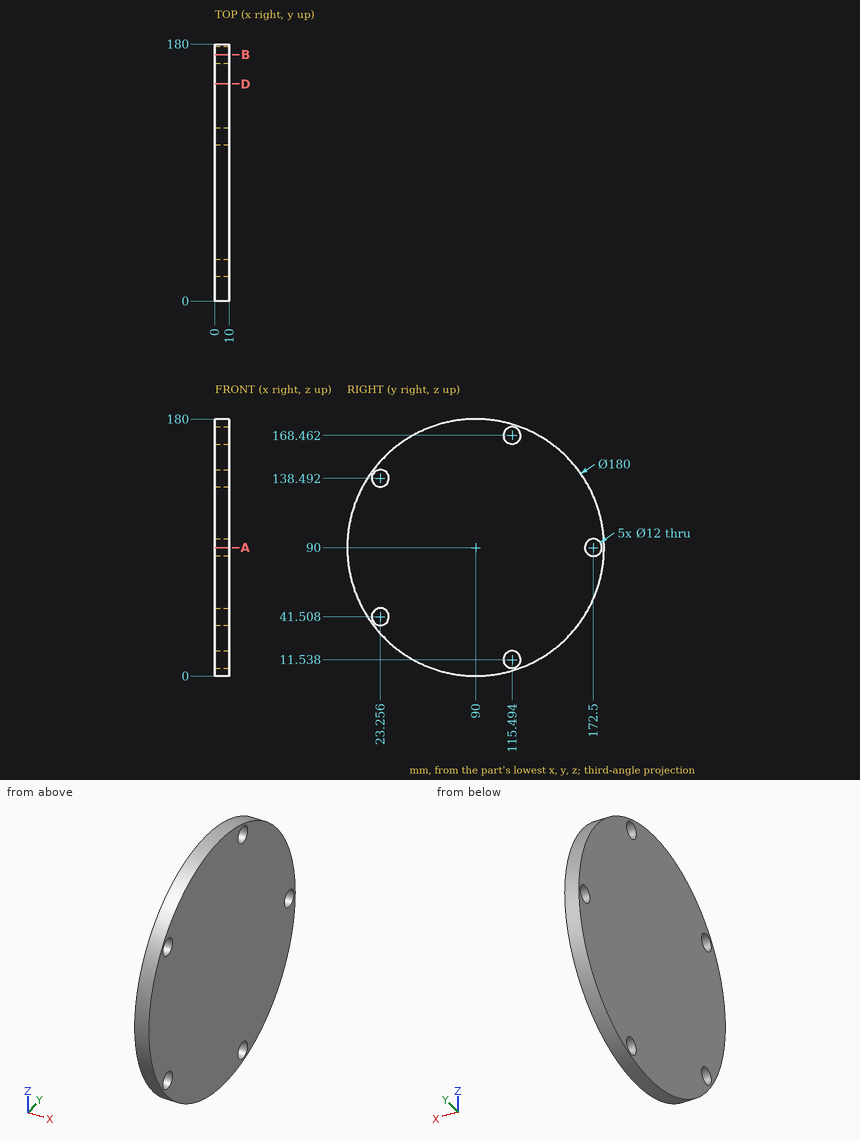
Design review of the part shown in the three views and the two pictorial views. Dimensions are in mm from the part's minimum x, y and z. Give positions to 0.01 mm unless a question says otherwise; leave off trailing zeros. Write each loop counter-clockwise with the first axis right and the second up, starting at its lowest first coordinate (ties: lowest second). Pieces come first, ordered by that corner, then holes. Notation, with made-up numbers: M 76.25,40.25 L 92.25,40.25 A10 ccw 92.25,51.25 Z; hole C 10,-39.5 d2. An arc over 180 degrees is marked long. Answer as CSV lines item,"result".
1. For pin 1 (4 mm diameter, centred on x = 4.5, z = 119, fed in from -Y) (1 decimal); pin 2 (11 mm diameter, centred on y = 172.5, z = 90, fed in from -X); pin 3 (6 mm diameter, centred on x = 2.5, z = 25, fed in from +Y); pin 4 (4 mm diameter, centred on x = 4.5, y = 99.5, fed in from -Z), all flat-tipped, find the tip position at first contact; note any pin that passes through.
Findings:
pin 1,"stops at y = 4.1"
pin 2,"passes through"
pin 3,"stops at y = 155.24"
pin 4,"stops at z = 0.31"
2. Consider section A-A, the plane z = 90. Write out the cut boundary in (x, y).
Findings:
outline,"M 0,0 L 10,0 L 10,166.5 L 0,166.5 Z; M 0,178.5 L 10,178.5 L 10,180 L 0,180 Z"
3. Wall thickness on line 1 (Z direction, x = 7, y = 112) (1 decimal); line 2 (Z direction, x = 8, y = 18) (1 decimal); line 3 (Y direction, x = 1, z = 39) (1 decimal): over which ranges is each line inside the solid? List them lowest first.
Findings:
line 1,"z = 2.7 to 6.7, 16.4 to 163.6, 173.3 to 177.3"
line 2,"z = 36 to 38.6, 44.4 to 135.6, 141.4 to 144"
line 3,"y = 15.8 to 17.8, 28.7 to 164.2"
4. Consider section D-D, the plane y = 152. Write out the cut boundary in (x, z).
Findings:
outline,"M 0,24.76 L 10,24.76 L 10,155.24 L 0,155.24 Z"
5. Consider section B-B, the plane y = 172.5. Write out the cut boundary in (x, z).
Findings:
outline,"M 0,54.03 L 10,54.03 L 10,84 L 0,84 Z; M 0,96 L 10,96 L 10,125.97 L 0,125.97 Z"
